```python
from build123d import *

# Parameters (mm, degrees)
SUSTAINER_TUBE_PROFILE_R   = 78.359
SUSTAINER_TUBE_PROFILE_R_2 = 76.2
SUSTAINER_TUBE_BODY_DEPTH  = 812.8
FIN_SLOT_CUT_REACH         = 833.471
FIN_SLOT_CUT_END_RADIUS    = 76.2
FIN_SLOT_PROFILE_W         = 2.54
FIN_SLOT_PROFILE_H         = 355.6
FIN_SLOT_PATTERN_COUNT     = 4


with BuildPart() as part:
    # Sustainer Tube Profile → Sustainer Tube Body (new body)
    with BuildSketch(Plane(origin=(0, 0, 0), x_dir=(1, 0, 0), z_dir=(0, 1, 0))):
        with Locations(Location((0, 0, 0), (0, 0, 270))):
            Circle(SUSTAINER_TUBE_PROFILE_R)
        with Locations(Location((0, 0, 0), (0, 0, 270))):
            Circle(SUSTAINER_TUBE_PROFILE_R_2, mode=Mode.SUBTRACT)
    extrude(amount=SUSTAINER_TUBE_BODY_DEPTH)

    # Fin Slot Cut: up to this cylinder (the profile starts outside it)
    fin_slot_cut_end = Plane(origin=(0, 212.471, 0), z_dir=(0, -1, 0)) * Cylinder(FIN_SLOT_CUT_END_RADIUS, 1820.342, mode=Mode.PRIVATE)
    # Fin Slot Profile → Fin Slot Cut (cut, up to the surface)
    with BuildSketch(Plane.XY.offset(78.359), mode=Mode.PRIVATE) as fin_slot_cut_sk1:
        with Locations((1.27, 212.471)):
            Rectangle(FIN_SLOT_PROFILE_W, FIN_SLOT_PROFILE_H)
    fin_slot_cut_tool1 = extrude(fin_slot_cut_sk1.sketch, amount=-FIN_SLOT_CUT_REACH, mode=Mode.PRIVATE) - fin_slot_cut_end
    # Fin Slot Profile → Fin Slot Cut (cut, up to the surface)
    with BuildSketch(Plane.XY.offset(78.359), mode=Mode.PRIVATE) as fin_slot_cut_sk2:
        with Locations((-1.27, 212.471)):
            Rectangle(FIN_SLOT_PROFILE_W, FIN_SLOT_PROFILE_H)
    fin_slot_cut_tool2 = extrude(fin_slot_cut_sk2.sketch, amount=-FIN_SLOT_CUT_REACH, mode=Mode.PRIVATE) - fin_slot_cut_end
    fin_slot_cut = fin_slot_cut_tool1.solids().sort_by_distance((1.27, 212.471, 78.359))[0] + fin_slot_cut_tool2.solids().sort_by_distance((-1.27, 212.471, 78.359))[0]
    add(fin_slot_cut, mode=Mode.SUBTRACT)

    # Fin Slot Pattern: Fin Slot Cut ×4 about axis
    fin_slot_pattern_axis = Axis((0, 0, 0), (0, 1, 0))
    for i in range(1, FIN_SLOT_PATTERN_COUNT):
        add(fin_slot_cut.rotate(fin_slot_pattern_axis, i * 360 / FIN_SLOT_PATTERN_COUNT), mode=Mode.SUBTRACT)


solid = part.part
```
Could you check a few things on this model? Use its own coordinates, in mm. Coordinates: 2 decimals unless noted, no trailing zeros. Order: outer loops, then holes, each group sorted by start corner. A loop starts at its lowest first (then second) coordinate and runs counter-clockwise, first axis right, second up. Notation, with made-up numbers: M -26,-17 L 13,-17 A20 cw 13,3 Z; hole C 81,-8 d11. An arc over 180 degrees is marked long. Use a Markdown table: item, result. Add a question column.
Q1. I want a section at B-B on x = 51.5. List the corners of the cut face in (y, z) for me.
Q2. I want a section at D-D on y = 683. List the corners of the cut face in (x, z) for me, then the cut area to 3 significant figures.
Q3. I want a section at C-C on z = -11. List the corners of the cut face in (x, y) for me.
Q4. I'm going to push flat-ended pins straight in: pin 1 (6 mm diameter, centred on x = 56, y = 708, fed in from -Z); pin 2 (5 mm diameter, centred on y = 249.5, z = 5, fed in from +X). Where does each tip first touch, or does it pass through?
Q5. I want a section at A-A on y = 61.5. List the corners of the cut face in (x, z) for me, then the cut area to 3 significant figures.
Q6. We'd pull the mould along X, two halves only. Please class faces 1 (the flat face through (-75, 0, 17)), 2 (the cylindrical face through (22.89, 400.71, 72.68)), 3 (the cylindrical face through (23.54, 400.71, 74.74)): pulls with the +X half, pulls with the -X half, needs draft (parallel to the pull), parting line crosses it, or undercut.
Q7. If I drill on L1, parallel to X at y = 244.5, z = 5; L2, parallel to X at y = 477, z = 0, over which ranges is the centre line in solid material (lowest first)?
Checked values:
| question | item | result |
|---|---|---|
| 1 | outline | M 0,-59.06 L 812.8,-59.06 L 812.8,-56.16 L 0,-56.16 Z; M 0,56.16 L 812.8,56.16 L 812.8,59.06 L 0,59.06 Z |
| 2 | outline | C 0,0 d156.72; hole C 0,0 d152.4 |
| 2 | area | 1,050 mm² |
| 3 | outline | M -77.58,0 L -75.4,0 L -75.4,812.8 L -77.58,812.8 Z; M 75.4,0 L 77.58,0 L 77.58,812.8 L 75.4,812.8 Z |
| 4 | pin 1 | z = -57.72 |
| 4 | pin 2 | x = 78.32 |
| 5 | outline | M -78.32,-2.54 A78.36 ccw -2.54,-78.32 L -2.54,-76.16 A76.2 cw -76.16,-2.54 Z; M -78.32,2.54 L -76.16,2.54 A76.2 cw -2.54,76.16 L -2.54,78.32 A78.36 ccw Z; M 2.54,-78.32 A78.36 ccw 78.32,-2.54 L 76.16,-2.54 A76.2 cw 2.54,-76.16 Z; M 2.54,76.16 A76.2 cw 76.16,2.54 L 78.32,2.54 A78.36 ccw 2.54,78.32 Z |
| 5 | area | 1,000 mm² |
| 6 | face 1 | needs draft |
| 6 | face 2 | undercut |
| 6 | face 3 | parting line crosses it |
| 7 | L1 | -78.2 to -76.04, 76.04 to 78.2 |
| 7 | L2 | -78.36 to -76.2, 76.2 to 78.36 |
